from build123d import *

# Parameters (mm, degrees)
F1_W      = 228.6
F1_H      = 76.2
F2_DEPTH  = 38.1
F3_W      = 76.2
F3_H      = 76.2
F4_DEPTH  = 76.2
F5_W      = 76.2
F5_H      = 76.2
F6_DEPTH  = 76.2
F7_W      = 76.2
F7_H      = 76.2
F8_DEPTH  = 152.4
F9_W      = 76.2
F9_H      = 76.2
F10_DEPTH = 76.2


# Not quite as in the source:
# - a variable given as a bare number and used for a length is read in inches; the dataset says mm whatever the document's units were


with BuildPart() as f2:
    # F1 (on Front) → F2 (new body, symmetric)
    with BuildSketch(Plane.XZ):
        Rectangle(F1_W, F1_H)
    extrude(amount=F2_DEPTH, both=True)

    # F3 (on face) → F4 (join)
    with BuildSketch(Plane.XZ.offset(38.1)):
        with Locations((76.2, 0)):
            Rectangle(F3_W, F3_H)
    extrude(amount=F4_DEPTH)

    # F5 (on face) → F6 (join)
    with BuildSketch(Plane(origin=(0, 38.1, 0), x_dir=(-1, 0, 0), z_dir=(0, 1, 0))):
        with Locations((76.2, 0)):
            Rectangle(F5_W, F5_H)
    extrude(amount=F6_DEPTH)

    # F7 (on face) → F8 (join)
    with BuildSketch(Plane.XY.offset(38.1)):
        with Locations((-76.2, 76.2)):
            Rectangle(F7_W, F7_H)
    extrude(amount=F8_DEPTH)

    # F9 (on face) → F10 (join)
    with BuildSketch(Plane.XZ.offset(-38.1)):
        with Locations((-76.2, 152.4)):
            Rectangle(F9_W, F9_H)
    extrude(amount=F10_DEPTH)


solid = f2.part
Here's how the part is built. I have some questions about the finished solid (model axes, mm). A direction names the side the tool comes from. Give positions to 0.01 mm unless a question says otherwise; leave off trailing zeros. Loops run counter-clockwise (first coordinate to the right, second up) from the corner with the lowest first, then second, coordinate; pieces in that order, holes last. Notation, with made-up numbers: (31, 10.5) -> (50, 10.5) arc R27 cw to (50, 39.5) -> close; hole circle Ø3 at (-29.75, 37). An arc over 180 degrees is marked (long way). Answer as a JSON object with one key per item and string values. Group by question number.
Item 1: Imagine slicing it at A-A on y = -34. Write out the boundary of the cut face in (x, z), then the cut area to 3 significant figures.
Item 2: On a 3-axis mill with a long thin cutter (end or side, diameter ignored), from which of +Z, -Z, +X, -X, +Y, -Y can I reach the whole of each face in a straight line? I mean faces 5 (the flat face through (37, 38.1, 1)), 6 (the flat face through (-77, 1, 114.3)), 7 (the flat face through (-39, -38.1, 1)). Say none if no direction works.
Item 3: Imagine slicing it at B-B on z = 21. Write out the boundary of the cut face in (x, y), then the cut area to 3 significant figures.
Item 4: Imagine slicing it at C-C on x = -88. Write out the boundary of the cut face in (y, z), then the cut area to 3 significant figures.
Item 5: I need wall thicknesses on L1, parallel to X at y = 55, z = 46; L2, parallel to Y at x = 52.5, z = 5; L3, parallel to Z at x = 38, y = 1. Which ranges of each line are inside material? Lowest first, please.
Item 6: Thinking about a two-plate mould opening in Z: for faces 1 (the flat face through (2, -2, -38.1)), 2 (the flat face through (-77, 39, 190.5)), 3 (the flat face through (-38.1, 56, 100)), 4 (the flat face through (-77, 38.1, 76)), which applies, pulls with the +Z half, pulls with the -Z half, needs draft (parallel to the pull), parting line crosses it, or undercut?
Item 7: Imagine slicing it at D-D on y = -88. Write out the boundary of the cut face in (x, z), then the cut area to 3 significant figures.
Answer list:
{
 "1": {"outline": "(-114.3, -38.1) -> (114.3, -38.1) -> (114.3, 38.1) -> (-114.3, 38.1) -> close; (-114.3, 114.3) -> (-38.1, 114.3) -> (-38.1, 190.5) -> (-114.3, 190.5) -> close", "area": "23,200 mm2"},
 "2": {"face 5": "+Z, -Z, +X, +Y", "face 6": "+X, -X, -Y", "face 7": "+Z, -Z, -X, -Y"},
 "3": {"outline": "(-114.3, -38.1) -> (38.1, -38.1) -> (38.1, -114.3) -> (114.3, -114.3) -> (114.3, 38.1) -> (-38.1, 38.1) -> (-38.1, 114.3) -> (-114.3, 114.3) -> close", "area": "29,000 mm2"},
 "4": {"outline": "(-38.1, -38.1) -> (114.3, -38.1) -> (114.3, 190.5) -> (-38.1, 190.5) -> (-38.1, 114.3) -> (38.1, 114.3) -> (38.1, 38.1) -> (-38.1, 38.1) -> close", "area": "29,000 mm2"},
 "5": {"L1": "x = -114.3 to -38.1", "L2": "y = -114.3 to 38.1", "L3": "z = -38.1 to 38.1"},
 "6": {"face 1": "pulls with the -Z half", "face 2": "pulls with the +Z half", "face 3": "needs draft", "face 4": "undercut"},
 "7": {"outline": "(38.1, -38.1) -> (114.3, -38.1) -> (114.3, 38.1) -> (38.1, 38.1) -> close", "area": "5,810 mm2"}
}
